```python
from build123d import *

# Parameters (mm, degrees)
SKETCH_1_R               = 10.5
EXTRUDE_1_DEPTH          = 10
EXTRUDE_START            = 3
SKETCH_3_R               = 17.5
EXTRUDE_1_2_DEPTH        = 3
SKETCH_4_R               = 1.5
SKETCH_4_R_2             = 3
CUT_EXTRUDE_1_DEPTH      = 28.955321497
CUT_EXTRUDE_2_REACH      = 34.504
CUT_EXTRUDE_2_END_RADIUS = 10.5
SKETCH_5_R               = 1.5


with BuildPart() as part:
    # 草图1 → Extrude 1 (new body)
    with BuildSketch(Plane.XY):
        Circle(SKETCH_1_R)
        with BuildLine():
            Line((-2, 8), (2, 8))
            Line((2, 8), (2, 5.656854249))
            ThreePointArc((2, 5.656854249), (0, -6), (-2, 5.656854249))
            Line((-2, 5.656854249), (-2, 8))
        make_face(mode=Mode.SUBTRACT)
    extrude(amount=EXTRUDE_1_DEPTH)

    # 草图3 → Extrude 1 2 (add)
    with BuildSketch(Plane(origin=(0, 0, 0), x_dir=(-1, 0, 0), z_dir=(0, 0, -1)).offset(EXTRUDE_START)):
        Circle(SKETCH_3_R)
        with BuildLine():
            Line((2, 8), (2, 5.656854249))
            ThreePointArc((2, 5.656854249), (0, -6), (-2, 5.656854249))
            Line((-2, 5.656854249), (-2, 8))
            Line((-2, 8), (2, 8))
        make_face(mode=Mode.SUBTRACT)
    extrude(amount=-EXTRUDE_1_2_DEPTH)

    # 草图4 → 切除-拉伸1 (cut, through all)
    with BuildSketch(Plane(origin=(0, 0, -3), x_dir=(-1, 0, 0), z_dir=(0, 0, -1))):
        with Locations((8.838834765, 8.838834765)):
            Circle(SKETCH_4_R)
        with Locations((-8.838834765, 8.838834765)):
            Circle(SKETCH_4_R_2)
        with Locations(Location((8.838834765, -8.838834765, 0), (0, 0, 92.166571934))):
            Circle(SKETCH_4_R_2)
        with Locations((-8.838834765, -8.838834765)):
            Circle(SKETCH_4_R)
    extrude(amount=-CUT_EXTRUDE_1_DEPTH, mode=Mode.SUBTRACT)

    # 切除-拉伸2: up to this cylinder (the profile starts inside it)
    cut_extrude_2_end = Plane(origin=(0, 0, 6), z_dir=(0, 0, -1)) * Cylinder(CUT_EXTRUDE_2_END_RADIUS, 91.008, mode=Mode.PRIVATE)
    # 草图5 → 切除-拉伸2 (cut, up to the surface)
    with BuildSketch(Plane.XZ.offset(-8), mode=Mode.PRIVATE) as cut_extrude_2_sk1:
        with Locations(Location((0, 6, 0), (0, 0, 270))):
            Circle(SKETCH_5_R)
    cut_extrude_2_tool1 = extrude(cut_extrude_2_sk1.sketch, amount=-CUT_EXTRUDE_2_REACH, mode=Mode.PRIVATE) & cut_extrude_2_end
    add(cut_extrude_2_tool1.solids().sort_by_distance((0, 8, 6))[0], mode=Mode.SUBTRACT)


solid = part.part
```
Geometry check sheet. Reference: the model listing, model coordinates, mm. A direction names the side the tool comes from. Give positions to 0.01 mm unless a question says otherwise; leave off trailing zeros. Order: outer loops, then holes, each group sorted by start corner. A loop starts at its lowest first (then second) coordinate and runs counter-clockwise, first axis right, second up. Notation, with made-up numbers: (38, -34.5) - (61, -34.5) arc R35 ccw to (61, -0.5) - close; hole circle Ø1 at (65, 50). An arc over 180 degrees is marked (long way). Write item = value, one per line. Start each with the question number.
1) Section check A-A (x = 0). Enter the section's corners in (y, z).
2) Section check C-C (z = 1.5). Enter the section's corners in (x, y), then the cut area to 3 significant figures.
3) Section check D-D (x = -6.5). Enter the section's corners in (y, z), then the cut area to 3 significant figures.
4) Scan lines: L1, parallel to Z at x = 0, y = 9.6; L2, parallel to X at y = 0, z = 8.5; L3, parallel to Y at x = 0, z = -1.55. Record each from-to range of solid material in increasing order.
5) Access from +Z, -Z, +X, -X, +Y, -Y to the whole of each face (thin tool, end or side, straight path). Record for faces 1 (the flat face through (-2, 7, 3)), 2 (the flat face through (0, -11, 0)), 3 (the cylindrical face through (0.07, 9.23, 7.5)).
6) Draft check along Y on faces 4 (the cylindrical face through (10.03, -9.75, -1.52)), 5 (the flat face through (5, -5, 10)), 6 (the cylindrical face through (6.068, 7.69, 0.52)), 7 (the cylindrical face through (-7.28, 7.566, 4.93)). Enter one of: released by +Y, released by -Y, zero draft, split by the parting line, or undercut.
7) Gauge pin test, flat ends, axial feed: pin 1 Ø5 at (x, y) = (-8.5, -9) entering from +Z; pin 2 Ø5 at (x, z) = (-10.5, 4) entering from +Y; pin 3 Ø4.5 at (x, z) = (-0.5, 4) entering from -Y; pin 4 Ø2 at (y, z) = (2.5, 6) entering from -X. Record the tip position at first contact, or that the pin passes through.
8) Section check B-B (z = -0.5). Enter the section's corners in (x, y), then the cut area to 3 significant figures.
Geometry check:
q1.outline = (-17.5, -3) - (-6, -3) - (-6, 10) - (-10.5, 10) - (-10.5, 0) - (-17.5, 0) - close; (8, -3) - (17.5, -3) - (17.5, 0) - (10.5, 0) - (10.5, 4.5) - (8, 4.5) - close; (8, 7.5) - (10.5, 7.5) - (10.5, 10) - (8, 10) - close
q2.outline = (-8.73, -5.84) arc R3 cw to (-5.84, -8.73) arc R10.5 ccw to (8.73, 5.84) arc R3 cw to (5.84, 8.73) arc R10.5 ccw to start; hole (-2, 5.66) arc R6 ccw (long way) to (2, 5.66) - (2, 8) - (-2, 8) - close
q2.area = 219 mm2
q3.outline = (-16.25, -3) - (-10.72, -3) - (-10.72, 0) - (-16.25, 0) - close; (-6.96, -3) - (16.25, -3) - (16.25, 0) - (8.25, 0) - (8.25, 10) - (-6.96, 10) - close
q3.area = 238 mm2
q4.L1 = -3 to 4.5, 7.5 to 10
q4.L2 = -10.5 to -6, 6 to 10.5
q4.L3 = -17.5 to -6, 8 to 17.5
q5.face_1 = +Z, -Z
q5.face_2 = +Z
q5.face_3 = +Y
q6.face_4 = undercut
q6.face_5 = zero draft
q6.face_6 = undercut
q6.face_7 = split by the parting line
q7.pin_1 = through
q7.pin_2 = 6.8
q7.pin_3 = -10.5
q7.pin_4 = -10.39
q8.outline = circle Ø35 at (0, 0); hole circle Ø6 at (-8.84, -8.84); hole circle Ø3 at (-8.84, 8.84); hole (-2, 5.66) arc R6 ccw (long way) to (2, 5.66) - (2, 8) - (-2, 8) - close; hole circle Ø6 at (8.84, 8.84); hole circle Ø3 at (8.84, -8.84)
q8.area = 770 mm2
